Here's how the part is built. I have some questions about the finished solid (model axes, mm). A direction names the side the tool comes from. Round coordinates to 2 decimals unless told otherwise and drop trailing zeros. Write each loop counter-clockwise with the first axis right and the second up, starting at its lowest first coordinate (ties: lowest second). Pieces come first, ordered by that corner, then holes. Notation, with made-up numbers: M 53,89.5 L 79,89.5 A26 cw 79,118.5 Z; hole C -39,6 d3. An arc over 180 degrees is marked long. Write item = value, one per line. Start each with the question number.
(1) If we mould it in two halves opening along X, with no side actions, what happens to faces 3 (the flat face through (0, 3, 5.08)), 4 (the cylindrical face through (-0.117, 2.504, -3.236)), 5 (the flat face through (-5.08, 3, 0))? For each: released by +X, released by -X, zero draft, split by the parting line, or undercut.
(2) I want a section at B-B (z = 0). List the corners of the cut face in (x, y) for me.
(3) I need wall thicknesses on line 1 along Z through (x, y) = (0, 2.5); line 2 along X through (y, z) = (1.65, 0); line 3 along Z through (x, y) = (-2.25, 3.35). Which ranges of each line are inside material? Lowest first, please.
(4) I want a section at C-C (y = 3.75). List the corners of the cut face in (x, z) for me, and give its area (3 significant figures).
(5) I want a section at A-A (x = 0). List the corners of the cut face in (y, z) for me.
(6) On a 3-axis mill with a long thin cutter (end or side, diameter ignored), from which of +Z, -Z, +X, -X, +Y, -Y can I reach the whole of each face in a straight line? I mean faces 1 (the flat face through (5.08, 3, 0)), 2 (the flat face through (0, 3, 2.73)). Say none if no direction works.
```python
from build123d import *

# Parameters (mm, degrees)
SKETCH1_W           = 10.16
SKETCH1_H           = 10.16
BOSS_EXTRUDE1_DEPTH = 5.08


with BuildPart() as part:
    # Sketch1 → Boss-Extrude1 (new body)
    with BuildSketch(Plane(origin=(0, 0, 0), x_dir=(1, 0, 0), z_dir=(0, 1, 0))):
        Rectangle(SKETCH1_W, SKETCH1_H)
        with BuildLine():
            Line((1.741336269, -2.7305), (-1.741336269, -2.7305))
            ThreePointArc((-1.741336269, -2.7305), (0, 3.2385), (1.741336269, -2.7305))
        make_face(mode=Mode.SUBTRACT)
    extrude(amount=BOSS_EXTRUDE1_DEPTH)


solid = part.part
```
Returned:
q1.face_3 = zero draft
q1.face_4 = undercut
q1.face_5 = released by -X
q2.outline = M -5.08,0 L -3.24,0 L -3.24,5.08 L -5.08,5.08 Z; M 3.24,0 L 5.08,0 L 5.08,5.08 L 3.24,5.08 Z
q3.line_1 = -5.08 to -3.24, 2.73 to 5.08
q3.line_2 = -5.08 to -3.24, 3.24 to 5.08
q3.line_3 = -5.08 to -2.33, 2.33 to 5.08
q4.outline = M -5.08,-5.08 L 5.08,-5.08 L 5.08,5.08 L -5.08,5.08 Z; hole M -1.74,2.73 A3.24 ccw long 1.74,2.73 Z
q4.area = 71.5 mm²
q5.outline = M 0,-5.08 L 5.08,-5.08 L 5.08,-3.24 L 0,-3.24 Z; M 0,2.73 L 5.08,2.73 L 5.08,5.08 L 0,5.08 Z
q6.face_1 = +Z, -Z, +X, +Y, -Y
q6.face_2 = +Y, -Y
